Check sheet for the modelled part. Datum: model origin and axes. Units: mm. Give positions to 0.01 mm unless a question says otherwise; leave off trailing zeros. Order: outer loops, then holes, each group sorted by start corner. A loop starts at its lowest first (then second) coordinate and runs counter-clockwise, first axis right, second up.
Autodesk Inventor part; units mm, degrees
ref_plane "YZ Plane" through (0, 0, 0) normal (1, 0, 0) x (0, 1, 0)
ref_plane "XZ Plane" through (0, 0, 0) normal (0, 1, 0) x (-1, 0, 0)
ref_plane "XY Plane" through (0, 0, 0) normal (0, 0, 1) x (1, 0, 0)
sketch "Sketch1" plane through (0, 0, 0) normal (0, 1, 0) x (-1, 0, 0)
  line L0 (135, 97.5) -> (-135, 97.5)
  line L1 (-135, 97.5) -> (-135, -97.5)
  line L2 (-135, -97.5) -> (135, -97.5)
  line L3 (135, -97.5) -> (135, 97.5)
  line L4 (135, 97.5) -> (-135, -97.5) construction
  line L5 (-135, 97.5) -> (135, -97.5) construction
  line L6 (135, 97.5) -> (-5, 97.5)
  line L7 (-5, 97.5) -> (-5, 109.5)
  line L8 (-5, 109.5) -> (135, 109.5)
  line L9 (135, 109.5) -> (135, 97.5)
  point P0 (0, 0)
  dimension "d0" = 270
  dimension "d1" = 195
  dimension "d2" = 140
  dimension "d3" = 12
  dimension "d4" = 0
  dimension "d5" = 0
extrude "Extrusion1" add sketch "Sketch1" along normal blind 2.5
sketch "Mounting Holes" plane through (0, 2.5, 0) normal (0, 1, 0) x (1, 0, 0)
  line L0 (-127, -88.9) -> (127, -88.9) construction
  line L1 (127, -88.9) -> (127, 88.9) construction
  line L2 (127, 88.9) -> (-127, 88.9) construction
  line L3 (-127, 88.9) -> (-127, -88.9) construction
  line L4 (-127, -88.9) -> (127, 88.9) construction
  line L5 (127, -88.9) -> (-127, 88.9) construction
  point P0 (0, 0)
  dimension "d32" = 254
  dimension "d33" = 177.8
hole "Hole3" at (-127, 2.5, -88.9) at (127, 2.5, -88.9) at (127, 2.5, 88.9) at (-127, 2.5, 88.9) direction (0, -1, 0) diameter 4.5 end through all
sketch "Cut" plane through (0, 2.5, 0) normal (0, 1, 0) x (1, 0, 0)
  line L0 (135, 80) -> (105, 80)
  line L1 (105, 80) -> (105, -80)
  line L2 (105, -80) -> (135, -80)
  line L3 (135, -80) -> (135, 80)
  line L4 (135, 80) -> (105, -80) construction
  line L5 (105, 80) -> (135, -80) construction
  line L6 (135, -97.5) -> (135, 97.5)
  line L7 (135, 97.5) -> (-135, 97.5)
  line L8 (-120, 10) -> (-135, 10)
  line L9 (-135, 10) -> (-135, -10)
  line L10 (-135, -10) -> (-120, -10)
  line L11 (-120, -10) -> (-120, 10)
  line L12 (-120, 10) -> (-135, -10) construction
  line L13 (-135, 10) -> (-120, -10) construction
  line L14 (-135, 97.5) -> (-135, -109.5)
  line L15 (135, 72.5) -> (135, 52.5)
  point P0 (0, 0)
  point P1 (120, 0)
  point P2 (-127.5, 0)
  dimension "d62" = 30
  dimension "d63" = 160
  dimension "d64" = 0
  dimension "d65" = 97.5
  dimension "d66" = 15
  dimension "d67" = 20
  dimension "d68" = 0
  dimension "d69" = 97.5
  dimension "d72" = 0
extrude "Plate-cutout" cut sketch "Cut" against normal through all
sketch "Sketch8" plane through (0, 2.5, 0) normal (0, 1, 0) x (1, 0, 0)
  line L0 (5, -109.5) -> (-135, -109.5) construction
  line L1 (-110, -109.5) -> (-110, 97.5) construction
  line L2 (135, 97.5) -> (-135, 97.5) construction
  line L3 (-135, 97.5) -> (-135, -109.5) construction
  line L4 (-135, 10) -> (-120, 10)
  line L5 (-120, -10) -> (-135, -10)
  point P0 (0, 0)
  point P1 (-110, 57.5)
  point P2 (-110, 32.5)
  dimension "d76" = 25
  dimension "d78" = 25
  dimension "d79" = 40
  dimension "d80" = 22.5
hole "Hole6" at (-110, 2.5, -57.5) at (-110, 2.5, -32.5) direction (0, -1, 0) diameter 2.459 end through all
sketch "Sketch9" plane through (0, 2.5, 0) normal (0, 1, 0) x (1, 0, 0)
  line L0 (-117, 12) -> (-82, 12) construction
  line L1 (-82, 12) -> (-82, 6.5) construction
  line L2 (-82, 6.5) -> (-117, 6.5) construction
  line L3 (-117, 6.5) -> (-117, 12) construction
  line L4 (-135, 97.5) -> (-135, -109.5)
  line L5 (-135, 97.5) -> (-135, -109.5)
  circle A0 centre (-110, 57.5) radius 1.2295
  point P0 (0, 0)
  point P1 (-135, 10)
  point P2 (-135, -10)
  dimension "d89" = 18
  dimension "d131" = 35
  dimension "d132" = 5.5
  dimension "d133" = 6.5
sketch "Sketch10" plane through (0, 2.5, 0) normal (0, 1, 0) x (1, 0, 0)
  line L0 (-17, 92.5) -> (49.04, 92.5) construction
  line L1 (49.04, 92.5) -> (49.04, 49.32) construction
  line L2 (49.04, 49.32) -> (-17, 49.32) construction
  line L3 (-17, 49.32) -> (-17, 92.5) construction
  line L4 (-17, 92.5) -> (49.04, 49.32) construction
  line L5 (49.04, 92.5) -> (-17, 49.32) construction
  line L6 (135, 97.5) -> (-135, 97.5)
  line L7 (-135, 97.5) -> (-135, -109.5)
  point P0 (0, 0)
  point P1 (16.02, 70.91)
  point P2 (-135, 10)
  dimension "d96" = 66.04
  dimension "d97" = 43.18
  dimension "d98" = 5
  dimension "d99" = 118
hole "B200 mini" at (-17, 2.5, -92.5) at (49.04, 2.5, -92.5) at (49.04, 2.5, -49.32) at (-17, 2.5, -49.32) direction (0, -1, 0) diameter 2.013 end through all
sketch "Sketch11" plane through (0, 2.5, 0) normal (0, 1, 0) x (1, 0, 0)
  line L0 (5, -109.5) -> (-135, -109.5) construction
  line L1 (-18, -109.5) -> (-18, 92.386) construction
  line L2 (-135, 97.5) -> (-135, -109.5) construction
  point P0 (0, 0)
  point P1 (-135, -10)
  point P2 (-18, -89.5)
  point P3 (-18, -31.5)
  point P4 (-110, -89.5)
  point P5 (-110, -31.5)
  dimension "d108" = 58
  dimension "d109" = 20
  dimension "d134" = 92
  dimension "d135" = 25
hole "RPI" at (-18, 2.5, 89.5) at (-18, 2.5, 31.5) at (-110, 2.5, 89.5) at (-110, 2.5, 31.5) direction (0, -1, 0) diameter 2.013 end through all
sketch "Sketch12" plane through (0, 2.5, 0) normal (0, 1, 0) x (1, 0, 0)
  line L0 (5, -97.5) -> (135, -97.5)
  line L1 (40, -97.5) -> (40, 97.2016) construction
  line L2 (-135, 97.5) -> (-135, -109.5) construction
  point P0 (0, 0)
  point P1 (40, 14.7)
  point P2 (40, -10.7)
  point P3 (40, -18.7)
  point P4 (40, -44.1)
  point P5 (40, -52.1)
  point P6 (40, -77.5)
  point P7 (-135, -10)
  dimension "d117" = 25.4
  dimension "d118" = 175
  dimension "d119" = 8
  dimension "d120" = 25.4
  dimension "d121" = 8
  dimension "d122" = 25.4
  dimension "d123" = 20
hole "Mini Circuits" at (40, 2.5, -14.7) at (40, 2.5, 10.7) at (40, 2.5, 18.7) at (40, 2.5, 44.1) at (40, 2.5, 52.1) at (40, 2.5, 77.5) direction (0, -1, 0) diameter 2.013 end through all
properties part number "Plate-1"
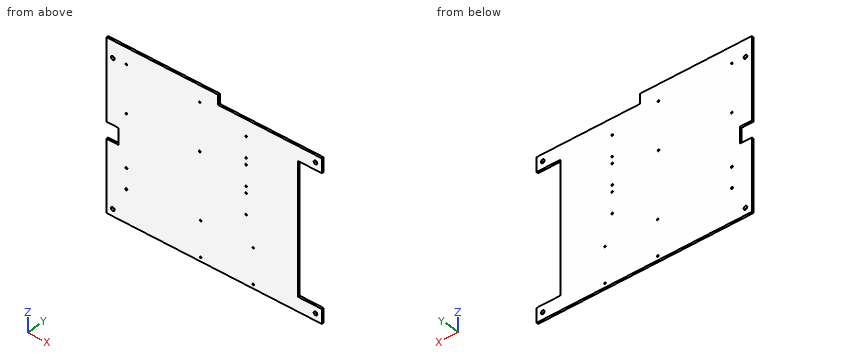
(1) Cross-section at B-B on z = 61.5. Enter the section's corners in (x, y), then the cut area to 3 significant figures.
Response values:
outline: (-135, 0) - (105, 0) - (105, 2.5) - (-135, 2.5) - close
area: 600 mm2
(2) Cross-section at A-A on y = 1.6. Count the separate pieces of the cut face and the enclosed holes in it, then the cut area to 3 significant figures.
Response values:
separate pieces: 1
enclosed holes: 20
area: 49,100 mm2
(3) Material ranges on L1, parallel to X at y = 1.45, z = -49.32; L2, parallel to X at y = 1.95, z = -88.9; L3, parallel to Z at x = -110, y = 1.2, recorded low to high.
Response values:
L1: x = -135 to -18.01, -15.99 to 48.03, 50.05 to 105
L2: x = -135 to -129.25, -124.75 to 124.75, 129.25 to 135
L3: z = -97.5 to -58.73, -56.27 to -33.73, -31.27 to 30.49, 32.51 to 88.49, 90.51 to 109.5
(4) Gauge pin test, flat ends, axial feed: pin 1 Ø2.5 at (x, z) = (40, 18.7) entering from +Y; pin 2 Ø1.6 at (x, z) = (-17, -92.5) entering from -Y; pin 3 Ø1.2 at (y, z) = (1.5, -2) entering from -X. Record the tip position at first contact, or that the pin passes through.
Response values:
pin 1: stops at y = 2.5
pin 2: passes through
pin 3: stops at x = -120
(5) Cross-section at C-C on x = 27. Enter the section's corners in (y, z).
Response values:
outline: (0, -97.5) - (2.5, -97.5) - (2.5, 97.5) - (0, 97.5) - close
